```python
from build123d import *

# Parameters (mm, degrees)
SKETCH1_W           = 5.6
SKETCH1_H           = 5.6
SKETCH1_R           = 0.75
BOSS_EXTRUDE1_DEPTH = 35
CUT_EXTRUDE1_DEPTH  = 36.555590278


with BuildPart() as part:
    # Sketch1 → Boss-Extrude1 (new body)
    with BuildSketch(Plane.XY):
        Rectangle(SKETCH1_W, SKETCH1_H)
        Circle(SKETCH1_R, mode=Mode.SUBTRACT)
    extrude(amount=BOSS_EXTRUDE1_DEPTH)

    # Sketch2 → Cut-Extrude1 (cut, through all)
    with BuildSketch(Plane.ZY.offset(2.8)):
        with BuildLine():
            Line((23, 1.5), (30, 1.5))
            ThreePointArc((30, 1.5), (31.5, 0), (30, -1.5))
            Line((30, -1.5), (23, -1.5))
            ThreePointArc((23, -1.5), (21.5, 0), (23, 1.5))
        make_face()
    extrude(amount=-CUT_EXTRUDE1_DEPTH, mode=Mode.SUBTRACT)


solid = part.part
```
Design review of the part built by this model. Coordinates are the model's own, in mm. A direction names the side the tool comes from. Give positions to 0.01 mm unless a question says otherwise; leave off trailing zeros. Write each loop counter-clockwise with the first axis right and the second up, starting at its lowest first coordinate (ties: lowest second). Pieces come first, ordered by that corner, then holes.
(1) Wall thickness on line 1 along X through (y, z) = (-0.05, 14); line 2 along Y through (x, z) = (1.9, 24): over which ranges is each line inside the solid? List them lowest first.
Checked values:
line 1: x = -2.8 to -0.75, 0.75 to 2.8
line 2: y = -2.8 to -1.5, 1.5 to 2.8
(2) Add section B-B (z = 26.5). Give the boundary of the cut face in (x, y), and give its area (3 significant figures).
Checked values:
outline: (-2.8, -2.8) - (2.8, -2.8) - (2.8, -1.5) - (-2.8, -1.5) - close; (-2.8, 1.5) - (2.8, 1.5) - (2.8, 2.8) - (-2.8, 2.8) - close
area: 14.6 mm2
(3) Add section A-A (x = 0). Give the boundary of the cut face in (y, z), and give its area (3 significant figures).
Checked values:
outline: (-2.8, 0) - (-0.75, 0) - (-0.75, 21.7) arc R1.5 cw to (-1.5, 23) - (-1.5, 30) arc R1.5 cw to (-0.75, 31.3) - (-0.75, 35) - (-2.8, 35) - close; (0.75, 0) - (2.8, 0) - (2.8, 35) - (0.75, 35) - (0.75, 31.3) arc R1.5 cw to (1.5, 30) - (1.5, 23) arc R1.5 cw to (0.75, 21.7) - close
area: 130 mm2
(4) Add section D-D (x = -1.5). Give the boundary of the cut face in (y, z).
Checked values:
outline: (-2.8, 0) - (2.8, 0) - (2.8, 35) - (-2.8, 35) - close; hole (-1.5, 23) arc R1.5 ccw to (1.5, 23) - (1.5, 30) arc R1.5 ccw to (-1.5, 30) - close
(5) Mouldability with a two-part tool opening along Y and no side actions: class faces 1 (the face through (-2.8, 0, 17)), 2 (the face through (0, 2.8, 17)), 3 (the face through (-0.039, 0.989, 31.128)) as +Y half, -Y half, draft (parallel to the pull), parting line (faces both ways), or undercut.
Checked values:
face 1: draft
face 2: +Y half
face 3: undercut
(6) Add section C-C (y = 0). Give the boundary of the cut face in (x, z), and give its area (4 significant figures).
Checked values:
outline: (-2.8, 0) - (-0.75, 0) - (-0.75, 21.5) - (-2.8, 21.5) - close; (-2.8, 31.5) - (-0.75, 31.5) - (-0.75, 35) - (-2.8, 35) - close; (0.75, 0) - (2.8, 0) - (2.8, 21.5) - (0.75, 21.5) - close; (0.75, 31.5) - (2.8, 31.5) - (2.8, 35) - (0.75, 35) - close
area: 102.5 mm2
(7) Tool access review of faces 4 (the face through (-0.039, -0.989, 21.872)), 5 (the face through (0, -2.8, 17)): name each direction out of +Z, -Z, +X, -X, +Y, -Y from which nothing blocks a thin tool from reaching the whole face with its end or side.
Checked values:
face 4: +X, -X
face 5: +Z, -Z, +X, -X, -Y
